Autodesk Inventor part; units mm, degrees
ref_plane "YZ Plane" through (0, 0, 0) normal (1, 0, 0) x (0, 1, 0)
ref_plane "XZ Plane" through (0, 0, 0) normal (0, 1, 0) x (-1, 0, 0)
ref_plane "XY Plane" through (0, 0, 0) normal (0, 0, 1) x (1, 0, 0)
sketch "Boceto1" plane through (0, 0, 0) normal (0, 1, 0) x (-1, 0, 0)
  line L0 (53, 63) -> (-53, 63)
  line L1 (-53, 63) -> (-53, -63)
  line L2 (-53, -63) -> (53, -63)
  line L3 (53, -63) -> (53, 63)
  point P0 (0, 0)
  point P1 (0, 63)
  dimension "d1" = 106
  dimension "d2" = 126
  dimension "d3" = 53
  dimension "d4" = 63
extrude "Extrusión1" add sketch "Boceto1" along normal blind 5
sketch "Boceto2" plane through (0, 5, 0) normal (0, 1, 0) x (1, 0, 0)
  circle A0 centre (-45.929, -42.384) radius 1.5
  line L0 (-53, -63) -> (53, -63)
  line L1 (-53, 63) -> (-53, -63)
  line L2 (-81, 0) -> (77, 0)
  line L3 (0, -130) -> (0, 128)
  circle A1 centre (-45.929, 42.384) radius 1.5
  line L4 (-53, -63) -> (-53, 63)
  circle A2 centre (45.929, -42.384) radius 1.5
  circle A3 centre (45.929, 42.384) radius 1.5
  point P0 (0, 0)
  dimension "d7" = 3
  dimension "d8" = 20.616
  dimension "d9" = 7.071
extrude "Extrusión2" add sketch "Boceto2" along normal blind 10 contours A0 | A1 | A2 | A3
sketch "Boceto3" plane through (0, 0, 0) normal (0, -1, 0) x (1, 0, 0)
  line L0 (-35, 52.5) -> (35, 52.5)
  line L1 (35, 52.5) -> (35, -52.5)
  line L2 (35, -52.5) -> (-35, -52.5)
  line L3 (-35, -52.5) -> (-35, 52.5)
  line L4 (53, -63) -> (-53, -63)
  line L5 (-53, 63) -> (53, 63)
  line L6 (53, 63) -> (53, -63)
  line L7 (-53, -63) -> (-53, 63)
  line L8 (35, 17.5) -> (-35, 17.5)
  line L9 (35, -17.5) -> (-35, -17.5)
  line L10 (0, 52.5) -> (0, -52.5)
  point P0 (0, 0)
  point P1 (0, 17.5)
  dimension "d12" = 52.5
  dimension "d13" = 126
  dimension "d14" = 106
  dimension "d15" = 52.5
  dimension "d16" = 35
  dimension "d17" = 35
  dimension "d18" = 35
  dimension "d19" = 35
  dimension "d20" = 35
extrude "Extrusión3" cut sketch "Boceto3" against normal blind 2 contours L0 L10 L8 L3 | L0 L1 L8 L10 | L8 L10 L9 L3 | L8 L1 L9 L10
properties part number "Tapa 0"
The listing builds one solid part. Answer for the finished solid, in the listing's coordinates (mm). A direction names the side the tool comes from. Coordinates: 2 decimals unless noted, no trailing zeros. Loops run counter-clockwise (first coordinate to the right, second up) from the corner with the lowest first, then second, coordinate; pieces in that order, holes last. Notation, with made-up numbers: (57.25, -33.5) - (74.25, -33.5) arc R11 cw to (74.25, -14.5) - close; hole circle Ø3 at (56.5, -16.75). An arc over 180 degrees is marked (long way). Use a Markdown table: item, result. Add a question column.
1) Find the intervals of material crossed by line 1 (X direction, y = 1.25, z = 39); line 2 (Y direction, x = 16.5, z = 33.5); line 3 (Y direction, x = 46, z = -31.5), in increasing order.
2) Given pin 1 (4 mm diameter, centred on x = 40.5, z = 7.5, fed in from +Y), flat-ended and moving along its own axis, determine where the tip first touches the part or whether it passes through.
3) The mould has two halves that part along X. Classify faces 1 (the cylindrical face through (46.621, 9.93, -43.715)), 2 (the flat face through (-46, 15, 42)), 3 (the flat face through (53, 2, 1)): released by +X, released by -X, zero draft, split by the parting line, or undercut.
4) For faces 4 (the flat face through (46, 15, 42)), 5 (the cylindrical face through (46.621, 9.93, 41.053)), 6 (the flat face through (0, 2, 18)), determine the directions among +Z, -Z, +X, -X, +Y, -Y from which every point of the face is accessible in a straight line to the end or side of a thin tool.
5) The part is cut by section C-C, the plane y = 11.25. Give the vertices of the cut face in (x, z), and give its area (3 significant figures).
6) The part is cut by section A-A, the plane z = 12. Give the vertices of the cut face in (x, y).
7) The part is cut by section D-D, the plane z = -36. Give the vertices of the cut face in (x, y), and give its area (3 significant figures).
8) The part is cut by section B-B, the plane x = 14. Give the vertices of the cut face in (y, z), and give its area (3 significant figures).
Here are the results:
| question | item | result |
|---|---|---|
| 1 | line 1 | x = -53 to -35, 35 to 53 |
| 1 | line 2 | y = 2 to 5 |
| 1 | line 3 | y = 0 to 5 |
| 2 | pin 1 | stops at y = 5 |
| 3 | face 1 | undercut |
| 3 | face 2 | zero draft |
| 3 | face 3 | released by +X |
| 4 | face 4 | +Z, -Z, +X, -X, +Y |
| 4 | face 5 | +Y |
| 4 | face 6 | -Y |
| 5 | outline | circle Ø3 at (-45.93, -42.38); circle Ø3 at (-45.93, 42.38); circle Ø3 at (45.93, -42.38); circle Ø3 at (45.93, 42.38) |
| 5 | area | 28.3 mm^2 |
| 6 | outline | (-53, 0) - (-35, 0) - (-35, 2) - (35, 2) - (35, 0) - (53, 0) - (53, 5) - (-53, 5) - close |
| 7 | outline | (-53, 0) - (53, 0) - (53, 5) - (-53, 5) - close |
| 7 | area | 530 mm^2 |
| 8 | outline | (0, -63) - (5, -63) - (5, 63) - (0, 63) - (0, 52.5) - (2, 52.5) - (2, -17.5) - (0, -17.5) - close |
| 8 | area | 490 mm^2 |
